Answer from the drawing. Dimensions are ordinates in mm from the lowest x, y and z of the part. Give positions to 0.01 mm unless a question says otherwise; leave off trailing zeros. Write each loop counter-clockwise with the first axis right and the second up, starting at its lowest first coordinate (ties: lowest second). Pieces come first, ordered by that corner, then holes.
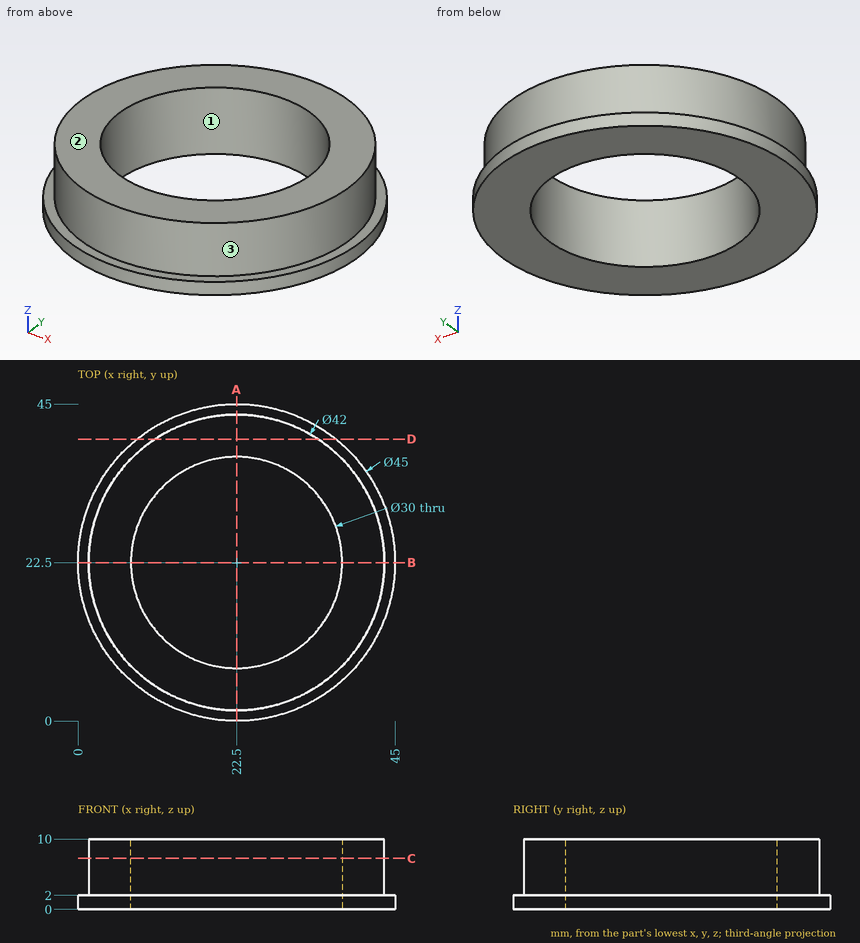
Item 1: Section D-D (y = 40) is taken. Write down the section's boundary in (x, z), and give its area (3 significant figures).
Result set:
outline: (8.36, 0) - (36.64, 0) - (36.64, 2) - (34.11, 2) - (34.11, 10) - (10.89, 10) - (10.89, 2) - (8.36, 2) - close
area: 242 mm2
Item 2: Determine the mould class of the marked faces 1, 2 and 3 for opening direction Y: pulls with the +Y half, pulls with the -Y half, needs draft (parallel to the pull), parting line crosses it, or undercut.
Result set:
face 1: undercut
face 2: needs draft
face 3: parting line crosses it
Item 3: Find the intervals of material crossed by line 1 along Y through (x, z) = (22.5, 7.75); line 2 along X through (y, z) = (30, 7.75); line 3 along X through (y, z) = (13, 4.75), in increasing order.
Result set:
line 1: y = 1.5 to 7.5, 37.5 to 43.5
line 2: x = 2.88 to 9.51, 35.49 to 42.12
line 3: x = 3.77 to 10.89, 34.11 to 41.23
Item 4: Each of these flat-tipped pins is pushed along its axis until it touches: pin 1 Ø4 at (x, z) = (20.5, 8.5) entering from -Y; pin 2 Ø3 at (y, z) = (16.5, 5.5) entering from -X; pin 3 Ø2 at (x, z) = (32, 7.5) entering from +Y; pin 4 Ø6 at (y, z) = (23, 3) entering from -X. Where does it stop, or does it pass through?
Result set:
pin 1: stops at y = 1.5
pin 2: stops at x = 1.99
pin 3: stops at y = 41.7
pin 4: stops at x = 0
Item 5: Section A-A (x = 22.5) is taken. Write down the section's boundary in (y, z).
Result set:
outline: (0, 0) - (7.5, 0) - (7.5, 10) - (1.5, 10) - (1.5, 2) - (0, 2) - close; (37.5, 0) - (45, 0) - (45, 2) - (43.5, 2) - (43.5, 10) - (37.5, 10) - close
Item 6: Section C-C (z = 7.25) is taken. Write down the section's boundary in (x, y), and give its area (3 significant figures).
Result set:
outline: circle Ø42 at (22.5, 22.5); hole circle Ø30 at (22.5, 22.5)
area: 679 mm2
